Print and shaded views of the part. All mm, measured from the part's lowest x, y and z. Round coordinates to 2 decimals unless told otherwise and drop trailing zeros. Loops run counter-clockwise (first coordinate to the right, second up) from the corner with the lowest first, then second, coordinate; pieces in that order, holes last. Notation, with made-up numbers: (81, 51) - (112, 51) arc R19 cw to (112, 80) - close; hole circle Ø6 at (47.25, 46). An arc over 180 degrees is marked (long way). Answer as a JSON object with one key per item and string values.
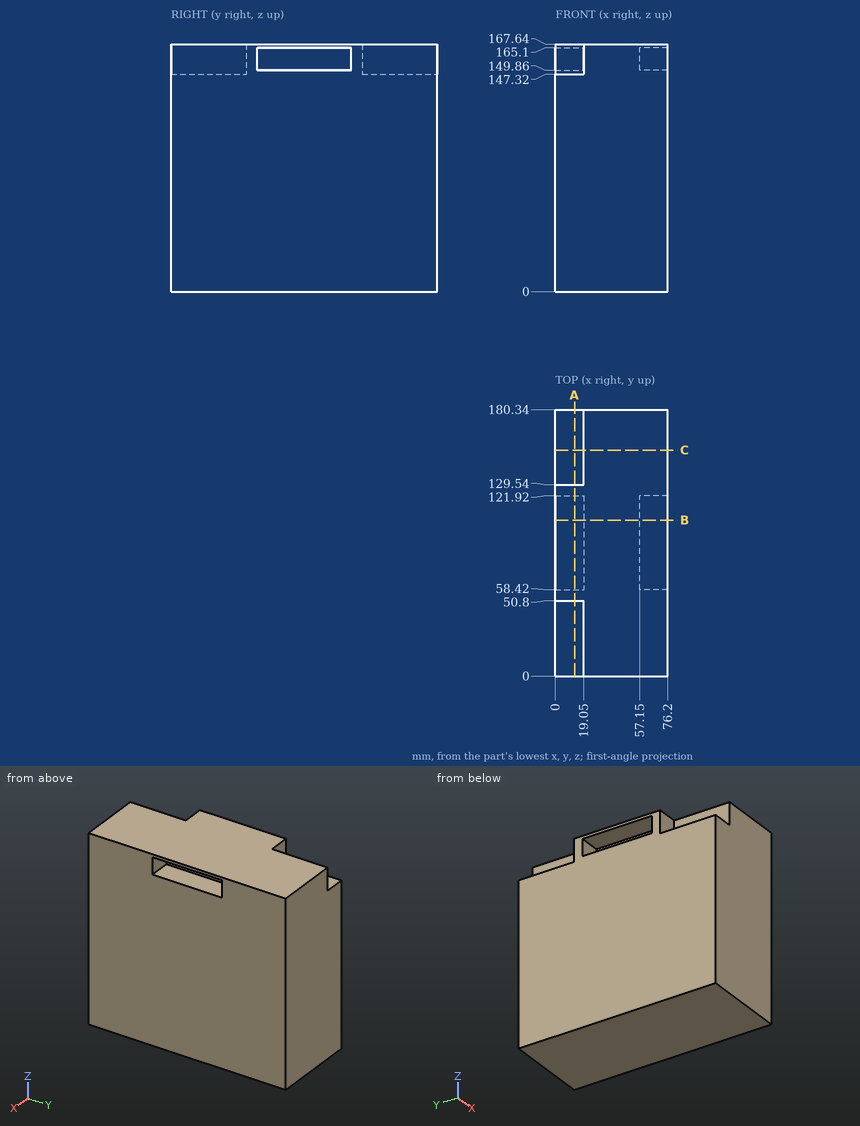
1) Slice it at B-B on y = 105.5. List the corners of the cut face in (x, z).
Values follow:
{"outline": "(0, 0) - (76.2, 0) - (76.2, 149.86) - (57.15, 149.86) - (57.15, 165.1) - (76.2, 165.1) - (76.2, 167.64) - (0, 167.64) - (0, 165.1) - (19.05, 165.1) - (19.05, 149.86) - (0, 149.86) - close"}
2) Probe probe 1 along Z at (x, y) = (10, 83); probe 2 along Z at (x, y) = (16, 21.5); probe 3 along Y at (x, z) = (7, 147.5). List the from-to ranges inside material, lowest first.
Values follow:
{"probe 1": "0 to 149.86, 165.1 to 167.64", "probe 2": "0 to 147.32", "probe 3": "50.8 to 129.54"}
3) Slice it at A-A on x = 13. List the corners of the cut face in (y, z), then the cut area to 3 significant figures.
Values follow:
{"outline": "(0, 0) - (180.34, 0) - (180.34, 147.32) - (129.54, 147.32) - (129.54, 167.64) - (50.8, 167.64) - (50.8, 147.32) - (0, 147.32) - close; hole (58.42, 149.86) - (121.92, 149.86) - (121.92, 165.1) - (58.42, 165.1) - close", "area": "27,200 mm²"}
4) Drop flat-ended pins along their axis: P1, Ø7.5, axis at y = 88, z = 158, coming from the +X side; P2, Ø21, axis at x = 13.5, z = 157.5, coming from the +Y side; P3, Ø7.5, axis at y = 89.5, z = 160, coming from the -X side; P4, Ø5.5, axis at x = 8.5, z = 161.5, coming from the -Y side. Give the stop position or say it passes through.
Values follow:
{"P1": "x = 57.15", "P2": "y = 180.34", "P3": "x = 19.05", "P4": "y = 50.8"}
5) Slice it at C-C on y = 153. List the corners of the cut face in (x, z).
Values follow:
{"outline": "(0, 0) - (76.2, 0) - (76.2, 167.64) - (19.05, 167.64) - (19.05, 147.32) - (0, 147.32) - close"}
